Autodesk Inventor part; units mm, degrees
ref_plane "YZ Plane" through (0, 0, 0) normal (1, 0, 0) x (0, 1, 0)
ref_plane "XZ Plane" through (0, 0, 0) normal (0, 1, 0) x (-1, 0, 0)
ref_plane "XY Plane" through (0, 0, 0) normal (0, 0, 1) x (1, 0, 0)
sketch "스케치1" plane through (0, 0, 0) normal (0, 1, 0) x (-1, 0, 0)
  line L0 (60, 80) -> (-60, 80)
  line L1 (-60, 80) -> (-60, -80)
  line L2 (-60, -80) -> (60, -80)
  line L3 (60, -80) -> (60, 80)
  line L4 (60, 80) -> (-60, -80) construction
  line L5 (-60, 80) -> (60, -80) construction
  point P0 (0, 0)
  dimension "d0" = 120
  dimension "d1" = 160
extrude "돌출1" add sketch "스케치1" along normal blind 60
sketch "스케치2" plane through (0, 60, 0) normal (0, 1, 0) x (1, 0, 0)
  line L0 (60, -80) -> (60, 80)
  line L1 (60, 80) -> (-60, 80)
  line L2 (55, 102.1646) -> (-55, 102.1646)
  line L3 (-55, 102.1646) -> (-55, -89.711)
  line L4 (-55, -89.711) -> (55, -89.711)
  line L5 (55, -89.711) -> (55, 102.1646)
  line L6 (-60, 80) -> (-60, -80)
  point P0 (0, 0)
  point P1 (55, 80)
  point P2 (-55, 80)
  dimension "d6" = 5
  dimension "d7" = 5
extrude "돌출2" cut sketch "스케치2" against normal blind 40 contours L5 L4 L3 L1
sketch "스케치12" plane through (60, 0, -80) normal (0, 0, -1) x (-1, 0, 0)
  line L0 (-34.8463, 10) -> (156.2634, 10)
  line L1 (156.2634, 10) -> (156.2634, -36.9465)
  line L2 (156.2634, -36.9465) -> (-34.8463, -36.9465)
  line L3 (-34.8463, -36.9465) -> (-34.8463, 10)
  line L4 (0, 0) -> (120, 0)
  point P0 (60, 0)
  dimension "d85" = 10
extrude "돌출10" cut sketch "스케치12" against normal through all
sketch "스케치13" plane through (-55, 20, 80) normal (0, 0, 1) x (1, 0, 0)
  line L0 (0, 40) -> (0, 0)
  line L1 (0, 0) -> (110, 0)
  line L2 (0, 40) -> (110, 40)
  line L3 (110, 40) -> (110, 0)
  line L4 (110, 0) -> (0, 0)
  line L5 (0, 0) -> (0, 40)
  point P0 (55, -20)
extrude "돌출11" add sketch "스케치13" against normal blind 5
sketch "스케치14" plane through (55, 20, -80) normal (0, 0, -1) x (-1, 0, 0)
  line L0 (0, 0) -> (0, 40)
  line L1 (110, 0) -> (0, 0)
  line L2 (0, 40) -> (110, 40)
  line L3 (110, 40) -> (110, 0)
  line L4 (110, 0) -> (0, 0)
  line L5 (0, 0) -> (0, 40)
  point P0 (55, -20)
extrude "돌출12" add sketch "스케치14" against normal blind 5
sketch "스케치15" plane through (60, 60, -80) normal (0, 0, -1) x (-1, 0, 0)
  point P0 (60, -60)
sketch "스케치16" plane through (60, 60, -80) normal (0, 0, -1) x (-1, 0, 0)
  point P0 (60, -60)
sketch "스케치17" plane through (0, 20, 0) normal (0, 1, 0) x (1, 0, 0)
  line L0 (7, 27) -> (45, 27)
  line L1 (45, 27) -> (45, 65)
  line L2 (45, 65) -> (7, 65)
  line L3 (7, 65) -> (7, 27)
  line L4 (55, 75) -> (55, -75)
  line L5 (55, 75) -> (-55, 75)
  circle A0 centre (7, 27) radius 1.6
  circle A1 centre (7, 65) radius 1.6
  circle A2 centre (45, 65) radius 1.6
  circle A3 centre (45, 27) radius 1.6
  line L6 (-47.9371, 14.7215) -> (-7.9371, 14.7215)
  line L7 (-7.9371, 14.7215) -> (-7.9371, 64.7215)
  line L8 (-7.9371, 64.7215) -> (-47.9371, 64.7215)
  line L9 (-47.9371, 64.7215) -> (-47.9371, 14.7215)
  point P0 (0, 0)
  dimension "d92" = 38
  dimension "d93" = 38
  dimension "d95" = 10
  dimension "d96" = 10
  dimension "d97" = 3.2
  dimension "d98" = 3.2
  dimension "d99" = 3.2
  dimension "d100" = 3.2
  dimension "d113" = 40
  dimension "d114" = 50
extrude "돌출13" cut sketch "스케치17" against normal through all contours L3 A0 L0 | L0 A0 L3 | A3 L1 L0 | L0 L1 A3 | A1 L2 L3 | L3 L2 A1 | A2 L2 L1 | L1 L2 A2
sketch "스케치19" plane through (60, 60, -80) normal (0, 0, -1) x (-1, 0, 0)
  line L0 (5, -40) -> (115, -40)
  circle A0 centre (46.5, -25) radius 8.5
  circle A1 centre (73.5, -25) radius 8.5
  line L1 (5, 0) -> (5, -40)
  line L2 (115, -40) -> (115, 0)
  point P0 (60, -60)
  dimension "d105" = 27
  dimension "d106" = 41.5
  dimension "d107" = 17
  dimension "d108" = 17
  dimension "d109" = 15
  dimension "d110" = 15
extrude "돌출14" cut sketch "스케치19" against normal through all
sketch "스케치21" plane through (0, 20, 0) normal (0, 1, 0) x (1, 0, 0)
  circle A0 centre (5.4243, 8.1678) radius 7.5
  line L0 (-49.3888, 17.2731) -> (-9.3888, 17.2731)
  line L1 (-9.3888, 17.2731) -> (-9.3888, 67.2731)
  line L2 (-9.3888, 67.2731) -> (-49.3888, 67.2731)
  line L3 (-49.3888, 67.2731) -> (-49.3888, 17.2731)
  point P0 (0, 0)
  dimension "d117" = 15
  dimension "d118" = 50
  dimension "d119" = 40
extrude "돌출15" cut sketch "스케치21" against normal through all contours A0
sketch "스케치23" plane through (0, 20, 0) normal (0, 1, 0) x (1, 0, 0)
  line L0 (-48.6, -65) -> (20, -65)
  line L1 (20, -65) -> (20, -11.6)
  line L2 (20, -11.6) -> (-48.6, -11.6)
  line L3 (-48.6, -11.6) -> (-48.6, -65)
  line L4 (55, 75) -> (55, -75)
  line L5 (-55, -75) -> (55, -75)
  circle A0 centre (4.7, -62.45) radius 1.6
  circle A1 centre (6.03, -14.15) radius 1.6
  circle A2 centre (-46.05, -47.16) radius 1.6
  circle A3 centre (-46.05, -19.23) radius 1.6
  point P0 (0, 0)
  dimension "d123" = 68.6
  dimension "d124" = 53.4
  dimension "d125" = 35
  dimension "d126" = 10
  dimension "d127" = 3.2
  dimension "d128" = 15.3
  dimension "d129" = 2.55
  dimension "d130" = 3.2
  dimension "d131" = 13.97
  dimension "d132" = 2.55
  dimension "d133" = 3.2
  dimension "d134" = 35.56
  dimension "d135" = 3.2
  dimension "d136" = 2.55
  dimension "d137" = 2.55
  dimension "d138" = 7.63
extrude "돌출16" cut sketch "스케치23" against normal through all contours A0 | A1 | A2 | A3
sketch "스케치24" plane through (0, 20, 0) normal (0, 1, 0) x (1, 0, 0)
  line L0 (-55, -75) -> (55, -75)
  line L1 (55, 75) -> (55, -75)
  line L2 (-55, -75) -> (55, -75)
  line L3 (55, -75) -> (55, 75)
  line L4 (55, 75) -> (-55, 75)
  line L5 (-55, 75) -> (-55, -75)
  point P0 (0, 0)
extrude "돌출17" cut sketch "스케치24" against normal through all
sketch "스케치25" plane through (0, 60, 0) normal (0, 1, 0) x (1, 0, 0)
  line L0 (-60, -80) -> (60, -80)
  line L1 (60, 80) -> (-60, 80)
  line L2 (-60, -80) -> (57, -80)
  line L3 (57, -80) -> (57, 80)
  line L4 (57, 80) -> (-60, 80)
  line L5 (-60, 80) -> (-60, -80)
  line L6 (60, -80) -> (60, 80)
  point P0 (0, 0)
  point P1 (57, -80)
  dimension "d143" = 3
extrude "돌출18" cut sketch "스케치25" against normal through all contours L5 L1 L3 L0
sketch "스케치26" plane through (60, 60, 80) normal (1, 0, 0) x (0, 0, -1)
  line L0 (64.5, 14.0975) -> (95.5, 14.0975)
  line L1 (95.5, 14.0975) -> (95.5, -3)
  line L2 (95.5, -3) -> (64.5, -3)
  line L3 (64.5, -3) -> (64.5, 14.0975)
  line L4 (160, -50) -> (160, 0)
  line L5 (0, 0) -> (160, 0)
  point P0 (80, -60)
  point P1 (95.5, 0)
  point P2 (64.5, 0)
  dimension "d146" = 31
  dimension "d147" = 64.5
  dimension "d148" = 3
extrude "돌출19" cut sketch "스케치26" against normal through all contours L5 L1 L2 L3
sketch "스케치27" plane through (60, 10, 80) normal (1, 0, 0) x (0, 0, -1)
  line L0 (65, 7.9616) -> (95, 7.9616)
  line L1 (95, 7.9616) -> (95, -3)
  line L2 (95, -3) -> (65, -3)
  line L3 (65, -3) -> (65, 7.9616)
  line L4 (160, 0) -> (160, 50)
  line L5 (0, 0) -> (160, 0)
  point P0 (80, -10)
  point P1 (95, 0)
  point P2 (65, 0)
  dimension "d151" = 30
  dimension "d152" = 65
  dimension "d153" = 3
extrude "돌출20" add sketch "스케치27" against normal blind 3 contours L5 L1 L2 L3
sketch "스케치28" plane through (60, 10, 80) normal (1, 0, 0) x (0, 0, -1)
  line L0 (157, 35.5) -> (165.4106, 35.5)
  line L1 (165.4106, 35.5) -> (165.4106, 14.5)
  line L2 (165.4106, 14.5) -> (157, 14.5)
  line L3 (157, 14.5) -> (157, 35.5)
  line L4 (95.5, 50) -> (160, 50)
  line L5 (160, 0) -> (160, 50)
  point P0 (80, -10)
  dimension "d156" = 21
  dimension "d157" = 14.5
  dimension "d160" = 3
extrude "돌출21" cut sketch "스케치28" against normal through all
mirror "미러3" about plane through (0, 0, 0) normal (0, 0, 1) of "돌출21"
sketch "스케치29" plane through (60, 60, -15.5) normal (1, 0, 0) x (0, 0, -1)
  point P0 (-15.5, -60)
properties part number "본체 겉면 레이저 옆판"
Input: part model. Units: mm. Frame: model coordinates. A direction names the side the tool comes from. Coordinates: 2 decimals unless noted, no trailing zeros. Write each loop counter-clockwise with the first axis right and the second up, starting at its lowest first coordinate (ties: lowest second). Pieces come first, ordered by that corner, then holes.
1) Section B-B on z = -1. Output: boundary loops of the cut face in (x, y).
2) Section C-C on y = 28.5. Output: boundary loops of the cut face in (x, z).
3) Material intervals for line 1 along Z through (x, y) = (59.7, 41); line 2 along Y through (x, z) = (58.2, -23.5); line 3 along Y through (x, z) = (57.8, -13), sorted ascending.
4) Mould query, pull axis Z, two halves, no side actions, for faces 4 (the flat face through (59, 60, 47)), 5 (the flat face through (59, 57, 0)), 6 (the flat face through (59, 17, -80)). Classes: pulls with the +Z half, pulls with the -Z half, needs draft (parallel to the pull), parting line crosses it, or undercut.
5) Set-up query: faces 1 (the flat face through (59, 24.5, -79)), 2 (the flat face through (59, 10, -48)), 3 (the flat face through (59, 58, 15.5)). Return all of +Z, -Z, +X, -X, +Y, -Y with unobstructed straight access to the full face (end or side cutting, diameter ignored); none if empty.
6) Pin query (flat end, axial travel): pin 1 Ø1.5 at (x, z) = (59, 79) entering from -Y; pin 2 Ø1.5 at (x, y) = (59, 33.5) entering from +Z; pin 3 Ø1.5 at (x, z) = (58, 2.5) entering from +Y. Return the tip coordinate at first contact, or that it passes through.
7) Section A-A on x = 58.1. Output: boundary loops of the cut face in (y, z), and give its area (3 significant figures).
Check result:
1. outline: (57, 7) - (60, 7) - (60, 57) - (57, 57) - close
2. outline: (57, -77) - (60, -77) - (60, 77) - (57, 77) - close
3. line 1: z = -77 to 77
3. line 2: y = 10 to 60
3. line 3: y = 7 to 57
4. face 4: needs draft
4. face 5: undercut
4. face 6: pulls with the -Z half
5. face 1: -Z, +X, -X
5. face 2: -Z, +X, -X, -Y
5. face 3: +X, -X, +Y
6. pin 1: stops at y = 10
6. pin 2: stops at z = 77
6. pin 3: stops at y = 57
7. outline: (7, -15) - (10, -15) - (10, -80) - (24.5, -80) - (24.5, -77) - (45.5, -77) - (45.5, -80) - (60, -80) - (60, -15.5) - (57, -15.5) - (57, 15.5) - (60, 15.5) - (60, 80) - (45.5, 80) - (45.5, 77) - (24.5, 77) - (24.5, 80) - (10, 80) - (10, 15) - (7, 15) - close
7. area: 7,870 mm2
